For this review, take the finished solid that the model builds, in its own axes (mm). A direction names the side the tool comes from. Coordinates: 2 decimals unless noted, no trailing zeros. Loops run counter-clockwise (first coordinate to the right, second up) from the corner with the lowest first, then second, coordinate; pieces in that order, holes last. Notation, with made-up numbers: (74.25, -28) -> (88.25, -28) arc R19 cw to (88.25, -20) -> close; hole circle Ø8 at (-32, 75.5). An arc over 180 degrees is marked (long way). Answer in a Markdown table with one row per item.
from build123d import *

# Parameters (mm, degrees)
F1_DEPTH = 66
F3_DEPTH = 25


with BuildPart() as f1:
    # F0 (on Top) → F1 (new body)
    with BuildSketch(Plane.XY):
        with BuildLine():
            Line((57.5, 0), (0, 0))
            Line((0, 0), (0, -2))
            Line((0, -2), (57.5, -2))
            ThreePointArc((57.5, -2), (59.62132, -2.87868), (60.5, -5))
            Line((60.5, -5), (60.5, -117))
            ThreePointArc((60.5, -117), (59.62132, -119.12132), (57.5, -120))
            Line((57.5, -120), (22.5, -120))
            Line((22.5, -120), (22.5, -122))
            Line((22.5, -122), (57.5, -122))
            ThreePointArc((57.5, -122), (61.035534, -120.535534), (62.5, -117))
            Line((62.5, -117), (62.5, -5))
            ThreePointArc((62.5, -5), (61.035534, -1.464466), (57.5, 0))
        make_face()
    extrude(amount=F1_DEPTH)

    # F2 (on face) → F3 (cut)
    with BuildSketch(Plane.XZ.offset(122)):
        with BuildLine():
            Line((34.5, 61.575), (29.5, 61.575))
            ThreePointArc((29.5, 61.575), (28.792893, 61.282107), (28.5, 60.575))
            Line((28.5, 60.575), (28.5, 5.425))
            ThreePointArc((28.5, 5.425), (28.792893, 4.717893), (29.5, 4.425))
            Line((29.5, 4.425), (34.5, 4.425))
            ThreePointArc((34.5, 4.425), (35.207107, 4.717893), (35.5, 5.425))
            Line((35.5, 5.425), (35.5, 60.575))
            ThreePointArc((35.5, 60.575), (35.207107, 61.282107), (34.5, 61.575))
        make_face()
    extrude(amount=-F3_DEPTH, mode=Mode.SUBTRACT)


solid = f1.part
Item 1: The part is to be moulded in two halves that separate along Y. For faces 1 (the flat face through (61, -34, 66)), 2 (the flat face through (44, -120, 33)), 3 (the cylindrical face through (61, -120.57, 32.54)), say which applies: +Y half, -Y half, draft (parallel to the pull), parting line (faces both ways), or undercut.
Worked answers:
| item | result |
|---|---|
| face 1 | draft |
| face 2 | undercut |
| face 3 | -Y half |
Item 2: Take a section at A-A, the plane x = 42. State the section outline as (y, z) points.
Worked answers:
| item | result |
|---|---|
| outline | (-122, 0) -> (-120, 0) -> (-120, 66) -> (-122, 66) -> close; (-2, 0) -> (0, 0) -> (0, 66) -> (-2, 66) -> close |
Item 3: Take a section at C-C, the plane x = 19. State the section outline as (y, z) points, and give its area (3 significant figures).
Worked answers:
| item | result |
|---|---|
| outline | (-2, 0) -> (0, 0) -> (0, 66) -> (-2, 66) -> close |
| area | 132 mm² |
Item 4: Insertion check: pin 1 (1 mm diameter, centred on y = -23.5, z = 44, fed in from -X); pin 2 (2 mm diameter, centred on y = -121, z = 30, fed in from +X); pin 3 (1 mm diameter, centred on y = -121.5, z = 48, fed in from -X). Each pin has a flat end and moves straight along its axis. Give the tip position at first contact, or say it passes through.
Worked answers:
| item | result |
|---|---|
| pin 1 | x = 60.5 |
| pin 2 | x = 61.5 |
| pin 3 | x = 22.5 |
Item 5: For faces 4 (the flat face through (28, -2, 33)), 5 (the flat face through (62.5, -62, 33)), list the 3-axis set-ups (+Z, -Z, +X, -X, +Y, -Y) from which the entire face can be reached by the end or side of a thin tool; tool diameter is ignored.
Worked answers:
| item | result |
|---|---|
| face 4 | +Z, -Z, -X |
| face 5 | +Z, -Z, +X, +Y, -Y |
Item 6: Take a section at D-D, the plane y = -74. State the section outline as (x, z) points.
Worked answers:
| item | result |
|---|---|
| outline | (60.5, 0) -> (62.5, 0) -> (62.5, 66) -> (60.5, 66) -> close |
Item 7: Take a section at B-B, the plane z = 47.5. State the section outline as (x, y) points, and give its area (3 significant figures).
Worked answers:
| item | result |
|---|---|
| outline | (0, -2) -> (57.5, -2) arc R3 cw to (60.5, -5) -> (60.5, -117) arc R3 cw to (57.5, -120) -> (35.5, -120) -> (35.5, -122) -> (57.5, -122) arc R5 ccw to (62.5, -117) -> (62.5, -5) arc R5 ccw to (57.5, 0) -> (0, 0) -> close; (22.5, -122) -> (28.5, -122) -> (28.5, -120) -> (22.5, -120) -> close |
| area | 420 mm² |
Item 8: For L1, parallel to Y at x = 23.5, z = 34.5; L2, parallel to X at y = -111.5, z = 41; L3, parallel to Y at x = 16, z = 7, list the stretches that pass through material, from the lowest coordinate up.
Worked answers:
| item | result |
|---|---|
| L1 | -122 to -120, -2 to 0 |
| L2 | 60.5 to 62.5 |
| L3 | -2 to 0 |
